from build123d import *

# Parameters (mm, degrees)
F1_DEPTH = 140


with BuildPart() as f1:
    # F0 (on Top) → F1 (new body)
    with BuildSketch(Plane.XY):
        with BuildLine():
            Line((-1.5, 0), (0, 0))
            Line((0, 0), (0, 85))
            ThreePointArc((0, 85), (4.564221, 89.980973), (9.924039, 85.868241))
            Line((9.924039, 85.868241), (22.679454, 13.528685))
            ThreePointArc((22.679454, 13.528685), (26.735252, 9.472887), (31.93362, 11.896926))
            Line((31.93362, 11.896926), (34.93362, 17.093079))
            Line((34.93362, 17.093079), (33.634582, 17.843079))
            Line((33.634582, 17.843079), (30.634582, 12.646926))
            ThreePointArc((30.634582, 12.646926), (26.995724, 10.950099), (24.156666, 13.789158))
            Line((24.156666, 13.789158), (11.40125, 86.128713))
            ThreePointArc((11.40125, 86.128713), (4.433488, 91.475266), (-1.5, 85))
            Line((-1.5, 85), (-1.5, 0))
        make_face()
    extrude(amount=F1_DEPTH)


solid = f1.part
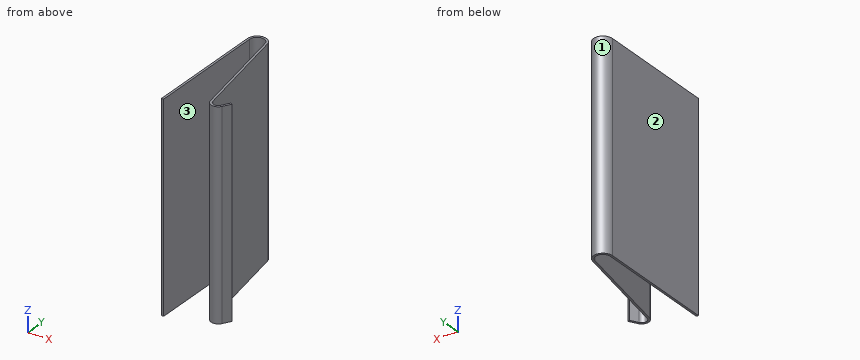
Model file for the job. Use its own axes, mm. Face numbers are marked on the shaded views. Round coordinates to 2 decimals unless told otherwise and drop trailing zeros. Loops run counter-clockwise (first coordinate to the right, second up) from the corner with the lowest first, then second, coordinate; pieces in that order, holes last. Notation, with made-up numbers: M 42,7.5 L 94,7.5 A17 ccw 94,13.5 Z; hole C 44,13 d3. An arc over 180 degrees is marked long. One line per question, with ' | ' between items.
1) Band-saw the part on C-C (y = 7.5). Give the cut face in (x, z), then the cut area to 3 significant figures.
Solved:
outline: M -1.5,0 L 0,0 L 0,140 L -1.5,140 Z | area: 210 mm²
2) Flat gauge pins, fed straight in: pin 1 (6 mm diameter, centred on x = 23.5, y = 26, fed in from +Z); pin 2 (8 mm diameter, centred on x = 6, y = 65, fed in from -Z); pin 3 (6 mm diameter, centred on x = 4.5, z = 35, fed in from -Y); pin 4 (8 mm diameter, centred on x = 31, z = 35.5, fed in from +Y). Where does each tip first touch, or does it go through?
Solved:
pin 1: stops at z = 140 | pin 2: passes through | pin 3: stops at y = 88.57 | pin 4: stops at y = 17.84
3) Band-saw the part on A-A (y = 40.5). Give the cut face in (x, z), then the cut area to 3 significant figures.
Solved:
outline: M -1.5,0 L 0,0 L 0,140 L -1.5,140 Z; M 17.92,0 L 19.45,0 L 19.45,140 L 17.92,140 Z | area: 423 mm²
4) Band-saw the part on B-B (z = 35.5). Give the cut face in (x, y), then the cut area to 3 significant figures.
Solved:
outline: M -1.5,0 L 0,0 L 0,85 A5 cw 9.92,85.87 L 22.68,13.53 A5 ccw 31.93,11.9 L 34.93,17.09 L 33.63,17.84 L 30.63,12.65 A3.5 cw 24.16,13.79 L 11.4,86.13 A6.5 ccw -1.5,85 Z | area: 288 mm²
5) Band-saw the part on D-D (x = 28). Give the cut face in (y, z).
Solved:
outline: M 9.41,0 L 10.92,0 L 10.92,140 L 9.41,140 Z
6) Mould opens along X. For the marked faces 1, 2 and 3 say: +X half, -X half, draft (parallel to the pull), parting line (faces both ways), or undercut.
Solved:
face 1: parting line | face 2: -X half | face 3: undercut
7) Drill centre lines: line 1 along X through (y, z) = (15, 40); line 2 along X through (y, z) = (17.5, 122.5); line 3 along X through (y, z) = (59, 45). Where is each one in solid material? Low to high.
Solved:
line 1: x = -1.5 to 0, 22.42 to 23.94, 31.99 to 33.73 | line 2: x = -1.5 to 0, 21.98 to 23.5, 33.44 to 34.23 | line 3: x = -1.5 to 0, 14.66 to 16.18
